```python
from build123d import *

# Parameters (mm, degrees)
F0_R     = 11.05
F0_R_2   = 4
F1_DEPTH = 7


with BuildPart() as f1:
    # F0 (on Top) → F1 (new body)
    with BuildSketch(Plane.XY):
        with BuildLine():
            ThreePointArc((-18.961918, 3.343498), (-20.777697, 1.23345), (-21.698821, -1.393503))
            ThreePointArc((-21.698821, -1.393503), (-36.856378, -21.27904), (-12.05622, -18.094979))
            ThreePointArc((-12.05622, -18.094979), (-9.320649, -18.610739), (-6.585405, -18.093251))
            ThreePointArc((-6.585405, -18.093251), (0, -22.00404), (6.585405, -18.093251))
            ThreePointArc((6.585405, -18.093251), (9.320649, -18.610739), (12.05622, -18.094979))
            ThreePointArc((12.05622, -18.094979), (36.856378, -21.27904), (21.698821, -1.393503))
            ThreePointArc((21.698821, -1.393503), (20.777697, 1.23345), (18.961918, 3.343498))
            ThreePointArc((18.961918, 3.343498), (19.056057, 11.00202), (12.376513, 14.749754))
            ThreePointArc((12.376513, 14.749754), (11.457048, 17.377288), (9.642601, 19.488482))
            ThreePointArc((9.642601, 19.488482), (0, 42.558079), (-9.642601, 19.488482))
            ThreePointArc((-9.642601, 19.488482), (-11.457048, 17.377288), (-12.376513, 14.749754))
            ThreePointArc((-12.376513, 14.749754), (-19.056057, 11.00202), (-18.961918, 3.343498))
        make_face()
        with Locations((-25.121734, -14.50404)):
            Circle(F0_R, mode=Mode.SUBTRACT)
        Polygon((-8.239777, -15.026816), (-8.454451, -13.536826), (-7.552666, -12.331446), (-6.062676, -12.116772), (-4.857296, -13.018557), (-4.642622, -14.508547), (-5.544407, -15.713927), (-7.034397, -15.928601), align=None, mode=Mode.SUBTRACT)
        with BuildLine():
            ThreePointArc((-17.783627, -1.417626), (-10.655181, -6.70699), (-10.402175, -15.579877))
            Line((-10.402175, -15.579877), (-17.783627, -1.417626))
        make_face(mode=Mode.SUBTRACT)
        Polygon((-15.243006, -0.317038), (-16.595347, -0.092157), (-17.392582, 1.023107), (-17.167701, 2.375449), (-16.052436, 3.172683), (-14.700095, 2.947802), (-13.90286, 1.832538), (-14.127741, 0.480197), align=None, mode=Mode.SUBTRACT)
        with Locations((0, -16.388141)):
            Circle(F0_R_2, mode=Mode.SUBTRACT)
        Polygon((7.896066, -13.042311), (8.377484, -14.325914), (7.810254, -15.573972), (6.526652, -16.055389), (5.278594, -15.488159), (4.797176, -14.204557), (5.364406, -12.956499), (6.648008, -12.475081), align=None, mode=Mode.SUBTRACT)
        with Locations((25.121734, -14.50404)):
            Circle(F0_R, mode=Mode.SUBTRACT)
        with BuildLine():
            ThreePointArc((10.119514, -14.69226), (11.136014, -5.874162), (18.693656, -1.218609))
            Line((18.693656, -1.218609), (10.119514, -14.69226))
        make_face(mode=Mode.SUBTRACT)
        with BuildLine():
            ThreePointArc((-11.049599, -0.09414), (-0.047071, 11.0499), (11.05, 0))
            ThreePointArc((11.05, 0), (0.047071, -11.0499), (-11.049599, -0.09414))
        make_face(mode=Mode.SUBTRACT)
        Polygon((17.133493, 0.377552), (15.95046, -0.553356), (14.455679, -0.375077), (13.524771, 0.807955), (13.703049, 2.302737), (14.886082, 3.233645), (16.380863, 3.055366), (17.311772, 1.872334), align=None, mode=Mode.SUBTRACT)
        with Locations((-14.450066, 8.117487)):
            Circle(F0_R_2, mode=Mode.SUBTRACT)
        Polygon((-7.49601, 14.090182), (-6.903013, 12.706524), (-7.462095, 11.308817), (-8.845753, 10.71582), (-10.243459, 11.274903), (-10.836456, 12.658561), (-10.277374, 14.056267), (-8.893716, 14.649264), align=None, mode=Mode.SUBTRACT)
        with BuildLine():
            ThreePointArc((7.664113, 16.109886), (-0.480834, 12.581152), (-8.291482, 16.798486))
            Line((-8.291482, 16.798486), (7.664113, 16.109886))
        make_face(mode=Mode.SUBTRACT)
        Polygon((10.641049, 13.679941), (10.773843, 12.315476), (9.902919, 11.256755), (8.538454, 11.123961), (7.479733, 11.994885), (7.34694, 13.35935), (8.217863, 14.418071), (9.582328, 14.550864), align=None, mode=Mode.SUBTRACT)
        with Locations((14.431565, 8.117487)):
            Circle(F0_R_2, mode=Mode.SUBTRACT)
        with Locations((0, 29.008079)):
            Circle(F0_R, mode=Mode.SUBTRACT)
    extrude(amount=F1_DEPTH)


solid = f1.part
```
Source: CAD feature listing. Evaluate the final solid. Frame: model axes, mm. A direction names the side the tool comes from. Coordinates: 2 decimals unless noted, no trailing zeros. Order: outer loops, then holes, each group sorted by start corner. A loop starts at its lowest first (then second) coordinate and runs counter-clockwise, first axis right, second up. Notation, with made-up numbers: (19, 72) - (70, 72) arc R23 cw to (70, 104) - close; hole circle Ø2 at (57, -14.5). An arc over 180 degrees is marked (long way). One line per item, written item: value.
1) Cut plane A-A on x = 27. Output: boundary loops of the cut face in (y, z), plus the area to 3 significant figures.
Computed values:
outline: (-27.92, 0) - (-25.39, 0) - (-25.39, 7) - (-27.92, 7) - close; (-3.61, 0) - (-1.08, 0) - (-1.08, 7) - (-3.61, 7) - close
area: 35.4 mm^2
2) Contact query for flat-ended pins moving along their axis: pin 1 (1.5 mm diameter, centred on x = 10.5, z = 4, fed in from +Y); pin 2 (7 mm diameter, centred on x = -14.45, y = 8.12, fed in from +Z); pin 3 (2 mm diameter, centred on x = -23.5, z = 5, fed in from +Y); pin 4 (2 mm diameter, centred on y = 30.5, z = 5.5, fed in from +X). Output: stop coordinate, or through.
Computed values:
pin 1: stops at y = 38.42
pin 2: passes through
pin 3: stops at y = -0.97
pin 4: stops at x = 13.54
3) Ray query, line 1 (Y direction, x = 25, z = 5); line 2 (X direction, y = -19, z = 4.5); line 3 (Y direction, x = -6, z = 1.5). Return the intervals inside material, ascending. Write a range as [from, to].
Computed values:
line 1: y = [-28.05, -25.55], [-3.45, -0.95]
line 2: x = [-37.9, -35.22], [-15.03, -12.34], [-6, -3.03], [3.03, 6], [12.34, 15.03], [35.22, 37.9]
line 3: y = [-19, -15.78], [-12.16, -9.28], [9.28, 14.5], [16.7, 19.73], [38.29, 41.16]
4) Reachability of faces 1 (the face through (-14.04, -8.6, 3.45)), 2 (the face through (-0.113, -22.003, 3.451)) from +Z, -Z, +X, -X, +Y, -Y: full face, straight path, thin tool, end or side. Return the list, or none.
Computed values:
face 1: +Z, -Z
face 2: +Z, -Z, -Y
5) Cut plane B-B on y = 27. Output: boundary loops of the cut face in (x, z), plus the area to 3 significant figures.
Computed values:
outline: (-13.4, 0) - (-10.87, 0) - (-10.87, 7) - (-13.4, 7) - close; (10.87, 0) - (13.4, 0) - (13.4, 7) - (10.87, 7) - close
area: 35.5 mm^2
6) Cut plane D-D on x = 0. Output: boundary loops of the cut face in (y, z), plus the area to 3 significant figures.
Computed values:
outline: (-22, 0) - (-20.39, 0) - (-20.39, 7) - (-22, 7) - close; (-12.39, 0) - (-11.05, 0) - (-11.05, 7) - (-12.39, 7) - close; (11.05, 0) - (12.57, 0) - (12.57, 7) - (11.05, 7) - close; (16.44, 0) - (17.96, 0) - (17.96, 7) - (16.44, 7) - close; (40.06, 0) - (42.56, 0) - (42.56, 7) - (40.06, 7) - close
area: 59.5 mm^2
7) Cut plane C-C on y = -8.5. Output: boundary loops of the cut face in (x, z), plus the area to 3 significant figures.
Computed values:
outline: (-37.27, 0) - (-34.4, 0) - (-34.4, 7) - (-37.27, 7) - close; (-15.85, 0) - (-14.09, 0) - (-14.09, 7) - (-15.85, 7) - close; (-9.93, 0) - (-7.06, 0) - (-7.06, 7) - (-9.93, 7) - close; (7.06, 0) - (9.95, 0) - (9.95, 7) - (7.06, 7) - close; (14.06, 0) - (15.85, 0) - (15.85, 7) - (14.06, 7) - close; (34.4, 0) - (37.27, 0) - (37.27, 7) - (34.4, 7) - close
area: 105 mm^2
8) Mould query, pull axis X, two halves, no side actions, for faces 3 (the face through (-12.6, 4.57, 3.45)), 4 (the face through (-6, 10, 0)). Classes: released by +X, released by -X, zero draft, split by the parting line, or undercut.
Computed values:
face 3: undercut
face 4: zero draft
